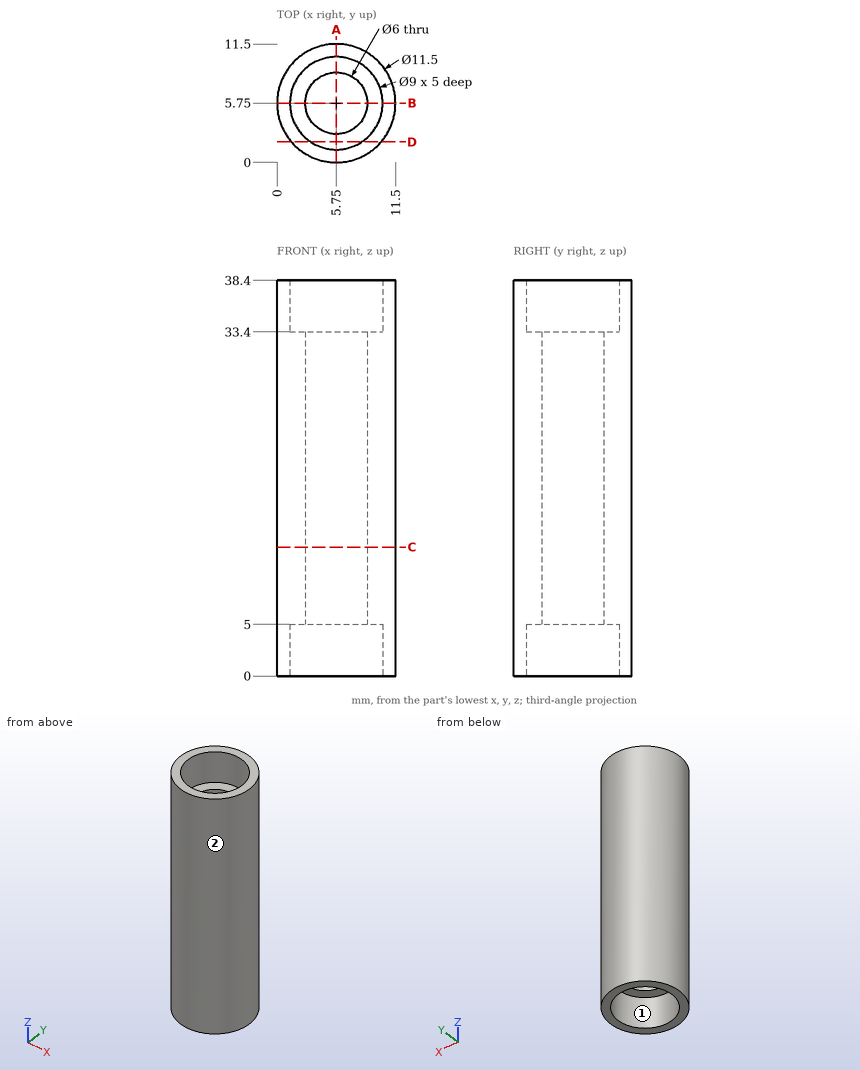
Could you check a few things on this drawing? It's one solid part, dimensions in mm from its lowest x, y, z. Coordinates: 2 decimals unless noted, no trailing zeros. Loops run counter-clockwise (first coordinate to the right, second up) from the corner with the lowest first, then second, coordinate; pieces in that order, holes last. Notation, with made-up numbers: (-36.5, 73) - (-26.5, 73) arc R7 cw to (-26.5, 82) - close; hole circle Ø4 at (71, 4). An arc over 180 degrees is marked (long way). Answer as a JSON object with one key per item and string values. Group by question number.
Item 1: If we section it at C-C (z = 12.5): List the corners of the cut face in (x, y) for me.
Item 2: If we section it at D-D (y = 2): List the corners of the cut face in (x, z) for me.
Item 3: If I drill on L1, parallel to Y at x = 5.75, z = 2.9; L2, parallel to Z at x = 3.75, y = 8.5; L3, parallel to Y at x = 5.75, z = 16.5, over which ranges is the centre line in solid material (lowest first)? Write a range as from..to.
Item 4: If we section it at A-A (x = 5.75): List the corners of the cut face in (y, z) for me, plus the area to 3 significant figures.
Item 5: If we mould it in two halves opening along X, with no side actions, what happens to the marked faces 1 and 2? For each: released by +X, released by -X, zero draft, split by the parting line, or undercut.
Item 6: For pin 1 (1 mm diameter, centred on x = 9, z = 28, fed in from +Y); pin 2 (4.5 mm diameter, centred on x = 5.5, y = 7, fed in from -Z); pin 3 (2 mm diameter, centred on y = 10, z = 18.5, fed in from +X); pin 4 (5.5 mm diameter, centred on x = 5.75, y = 5.75, fed in from -Z), each with a flat end and sliding along its axis, tell me the tip position at first contact or that it passes through.
Returned:
{
 "1": {"outline": "circle Ø11.5 at (5.75, 5.75); hole circle Ø6 at (5.75, 5.75)"},
 "2": {"outline": "(1.39, 0) - (3.26, 0) - (3.26, 5) - (8.24, 5) - (8.24, 0) - (10.11, 0) - (10.11, 38.4) - (8.24, 38.4) - (8.24, 33.4) - (3.26, 33.4) - (3.26, 38.4) - (1.39, 38.4) - close"},
 "3": {"L1": "y = 0..1.25, 10.25..11.5", "L2": "z = 5..33.4", "L3": "y = 0..2.75, 8.75..11.5"},
 "4": {"outline": "(0, 0) - (1.25, 0) - (1.25, 5) - (2.75, 5) - (2.75, 33.4) - (1.25, 33.4) - (1.25, 38.4) - (0, 38.4) - close; (8.75, 5) - (10.25, 5) - (10.25, 0) - (11.5, 0) - (11.5, 38.4) - (10.25, 38.4) - (10.25, 33.4) - (8.75, 33.4) - close", "area": "181 mm²"},
 "5": {"face 1": "undercut", "face 2": "split by the parting line"},
 "6": {"pin 1": "stops at y = 10.8", "pin 2": "stops at z = 5", "pin 3": "stops at x = 10.49", "pin 4": "passes through"}
}
